```python
from build123d import *

# Parameters (mm, degrees)
SKETCH_1_R          = 15
SKETCH_1_R_2        = 1.5
SKETCH_1_R_3        = 3
EXTRUDE_1_DEPTH     = 3
SKETCH_2_R          = 1.5
SKETCH_2_R_2        = 3
EXTRUDE_2_DEPTH     = 5
SKETCH_5_R          = 2.6
CUT_EXTRUDE_1_DEPTH = 3
EXTRUDE_3_DEPTH     = 15
FILLET_5_R          = 1
FILLET_6_R          = 1
FILLET_7_R          = 3


with BuildPart() as part:
    # 草图1 → 凸台-拉伸1 (new body)
    with BuildSketch(Plane(origin=(0, 0, 0), x_dir=(1, 0, 0), z_dir=(0, 1, 0))):
        with Locations(Location((0, 0, 0), (0, 0, 270))):
            Circle(SKETCH_1_R)
        with Locations(Location((0, 7, 0), (0, 0, 270))):
            Circle(SKETCH_1_R_2, mode=Mode.SUBTRACT)
        with Locations(Location((4.949747468, 4.949747468, 0), (0, 0, 270))):
            Circle(SKETCH_1_R_2, mode=Mode.SUBTRACT)
        with Locations(Location((7, 0, 0), (0, 0, 270))):
            Circle(SKETCH_1_R_2, mode=Mode.SUBTRACT)
        with Locations(Location((4.949747468, -4.949747468, 0), (0, 0, 270))):
            Circle(SKETCH_1_R_2, mode=Mode.SUBTRACT)
        with Locations(Location((0, -7, 0), (0, 0, 270))):
            Circle(SKETCH_1_R_2, mode=Mode.SUBTRACT)
        with Locations(Location((-4.949747468, -4.949747468, 0), (0, 0, 270))):
            Circle(SKETCH_1_R_2, mode=Mode.SUBTRACT)
        with Locations(Location((-7, 0, 0), (0, 0, 270))):
            Circle(SKETCH_1_R_2, mode=Mode.SUBTRACT)
        with Locations(Location((-4.949747468, 4.949747468, 0), (0, 0, 270))):
            Circle(SKETCH_1_R_2, mode=Mode.SUBTRACT)
        with Locations(Location((0, 0, 0), (0, 0, 270))):
            Circle(SKETCH_1_R_3, mode=Mode.SUBTRACT)
    extrude(amount=EXTRUDE_1_DEPTH)

    # 草图2 → 凸台-拉伸2 (add)
    with BuildSketch(Plane(origin=(0, 3, 0), x_dir=(1, 0, 0), z_dir=(0, 1, 0))):
        with BuildLine():
            ThreePointArc((34.287340692, 7.026967216), (22.116276452, 66.414383351), (-23.229202466, 26.18022446))
            ThreePointArc((-23.229202466, 26.18022446), (-68.574681385, -14.053934431), (-11.058138226, -33.207191676))
            ThreePointArc((-11.058138226, -33.207191676), (46.458404933, -52.36044892), (34.287340692, 7.026967216))
        make_face()
        with Locations(Location((-4.949747468, 4.949747468, 0), (0, 0, 270))):
            Circle(SKETCH_2_R, mode=Mode.SUBTRACT)
        with Locations(Location((-4.949747468, -4.949747468, 0), (0, 0, 270))):
            Circle(SKETCH_2_R, mode=Mode.SUBTRACT)
        with Locations(Location((0, -7, 0), (0, 0, 270))):
            Circle(SKETCH_2_R, mode=Mode.SUBTRACT)
        with Locations(Location((0, 0, 0), (0, 0, 270))):
            Circle(SKETCH_2_R_2, mode=Mode.SUBTRACT)
        with Locations(Location((-7, 0, 0), (0, 0, 270))):
            Circle(SKETCH_2_R, mode=Mode.SUBTRACT)
        with Locations(Location((4.949747468, -4.949747468, 0), (0, 0, 270))):
            Circle(SKETCH_2_R, mode=Mode.SUBTRACT)
        with Locations(Location((7, 0, 0), (0, 0, 270))):
            Circle(SKETCH_2_R, mode=Mode.SUBTRACT)
        with Locations(Location((4.949747468, 4.949747468, 0), (0, 0, 270))):
            Circle(SKETCH_2_R, mode=Mode.SUBTRACT)
        with Locations(Location((0, 7, 0), (0, 0, 270))):
            Circle(SKETCH_2_R, mode=Mode.SUBTRACT)
    extrude(amount=EXTRUDE_2_DEPTH)

    # 草图5 → 切除-拉伸1 (cut)
    with BuildSketch(Plane(origin=(0, 8, 0), x_dir=(1, 0, 0), z_dir=(0, 1, 0))):
        with Locations(Location((0, 7, 0), (0, 0, 270))):
            Circle(SKETCH_5_R)
        with Locations(Location((4.949747468, 4.949747468, 0), (0, 0, 270))):
            Circle(SKETCH_5_R)
        with Locations(Location((7, 0, 0), (0, 0, 270))):
            Circle(SKETCH_5_R)
        with Locations(Location((4.949747468, -4.949747468, 0), (0, 0, 270))):
            Circle(SKETCH_5_R)
        with Locations(Location((0, -7, 0), (0, 0, 270))):
            Circle(SKETCH_5_R)
        with Locations(Location((-4.949747468, -4.949747468, 0), (0, 0, 270))):
            Circle(SKETCH_5_R)
        with Locations(Location((-7, 0, 0), (0, 0, 270))):
            Circle(SKETCH_5_R)
        with Locations(Location((-4.949747468, 4.949747468, 0), (0, 0, 270))):
            Circle(SKETCH_5_R)
    extrude(amount=-CUT_EXTRUDE_1_DEPTH, mode=Mode.SUBTRACT)

    # 草图3 → 凸台-拉伸3 (add)
    with BuildSketch(Plane(origin=(0, 8, 0), x_dir=(1, 0, 0), z_dir=(0, 1, 0))):
        with BuildLine():
            ThreePointArc((34.287340692, 7.026967216), (22.116276452, 66.414383351), (-23.229202466, 26.18022446))
            ThreePointArc((-23.229202466, 26.18022446), (-68.574681385, -14.053934431), (-11.058138226, -33.207191676))
            ThreePointArc((-11.058138226, -33.207191676), (46.458404933, -52.36044892), (34.287340692, 7.026967216))
        make_face()
        with BuildLine():
            ThreePointArc((31.118546415, 6.377543462), (21.642356242, 64.991217994), (-21.08238786, 23.760679994))
            ThreePointArc((-21.08238786, 23.760679994), (-67.105223926, -13.752778694), (-10.036158556, -30.138223456))
            ThreePointArc((-10.036158556, -30.138223456), (45.462867684, -51.2384393), (31.118546415, 6.377543462))
        make_face(mode=Mode.SUBTRACT)
    extrude(amount=EXTRUDE_3_DEPTH)

    # 圆角5
    fillet_5_edges = [part.edges().sort_by_distance(p)[0] for p in [
        (31.118546415, 15.5, -6.377543462),
        (-21.08238786, 15.5, -23.760679994),
        (-10.036158556, 15.5, 30.138223456),
    ]]
    fillet(fillet_5_edges, radius=FILLET_5_R)

    # 圆角6
    fillet_6_edges = [part.edges().sort_by_distance(p)[0] for p in [
        (-67.105223926, 23, 13.752778694),
        (45.462867684, 23, 51.2384393),
        (21.642356242, 23, -64.991217994),
        (-21.886725168, 23, -24.667199764),
        (32.30578422, 23, -6.620860119),
        (-10.419059052, 23, 31.288059883),
    ]]
    fillet(fillet_6_edges, radius=FILLET_6_R - 0.0004)  # a hair under: the kernel refuses the full size

    # 圆角7
    fillet_7_edges = [part.edges().sort_by_distance(p)[0] for p in [
        (-11.058138226, 13, 33.207191676),
        (34.287340692, 13, -7.026967216),
        (-23.229202466, 13, -26.18022446),
    ]]
    fillet(fillet_7_edges, radius=FILLET_7_R)


solid = part.part
```
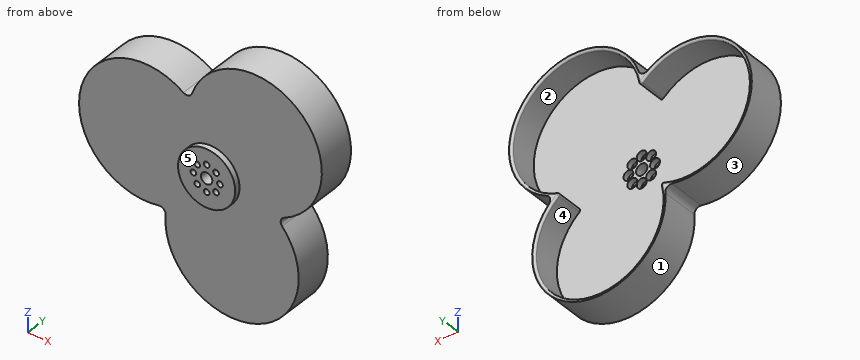
CAD build for the part. Positions are in the model's coordinates, mm. Face numbers are marked on the shaded views. A direction names the side the tool comes from. Give positions to 0.01 mm unless a question says otherwise; leave off trailing zeros. Use one line per item in the form item = value.
Item 1: Two-plate mould, pull along Z, no slides. Class the marked faces 3, 4 and 5: pulls with the +Z half, pulls with the -Z half, needs draft (parallel to the pull), parting line crosses it, or undercut.
Determined:
face_3 = parting line crosses it
face_4 = undercut
face_5 = needs draft
Item 2: Which spindle directions (+Z, -Z, +X, -X, +Y, -Y) get a long thin tool onto all of the face, cutting with end or side? Do the marked faces 1 and 2. Say none if no direction does.
Determined:
face_1 = +Y, -Y
face_2 = +Y
Item 3: Slice it at A-A (x = 0). Count the separate pieces of the cut face and the enclosed holes in it, plus the area to 3 significant figures.
Determined:
separate_pieces = 4
enclosed_holes = 0
area = 629 mm2
Item 4: Flat gauge pins, fed straight in: pin 1 (1 mm diameter, centred on x = -7.5, y = 7, fed in from -Z); pin 2 (2 mm diameter, centred on y = 6, z = 5, fed in from +X); pin 3 (5.5 mm diameter, centred on x = -6, z = -5, fed in from +Y). Where does each tip first touch, or does it go through?
Determined:
pin_1 = -63.19
pin_2 = 51.83
pin_3 = 8
Item 5: Drill centre lines: probe 1 along X at (y, z) = (7.2, -7); probe 2 along Z at (x, y) = (-4, 1.25); probe 3 along Y at (x, z) = (-54.5, 33). Where is each one in solid material? Low to high. Write a range as from..to.
Determined:
probe_1 = -66.35..-6.55, -3.35..-2.6, 2.6..3.35, 6.55..36.81
probe_2 = -14.46..-6.11, -3.79..3.79, 6.11..14.46
probe_3 = 3..8
